Work out the finished part from the listing and answer in its coordinate system (mm). Round coordinates to 2 decimals unless told otherwise and drop trailing zeros. Order: outer loops, then holes, each group sorted by start corner. A loop starts at its lowest first (then second) coordinate and runs counter-clockwise, first axis right, second up. Notation, with made-up numbers: (-35.75, 38) - (1.25, 38) arc R31 ccw to (1.25, 70) - close; hole circle Ø10 at (74.5, 21). An arc over 180 degrees is marked (long way). Answer in a Markdown table with one row per item.
from build123d import *

# Parameters (mm, degrees)
SKETCH_1_W      = 32
SKETCH_1_H      = 10
SKETCH_1_R      = 1.25
EXTRUDE_1_DEPTH = 18
SKETCH_4_W      = 32
SKETCH_4_H      = 10
SKETCH_4_R      = 1.25
EXTRUDE_3_DEPTH = 1
FILLET_3_R      = 5
FILLET_4_R      = 5


with BuildPart() as part:
    # 草图1 → 凸台-拉伸1 (new body)
    with BuildSketch(Plane(origin=(0, 0, 0), x_dir=(1, 0, 0), z_dir=(0, 1, 0))):
        with Locations((16, 5)):
            Rectangle(SKETCH_1_W, SKETCH_1_H)
        with Locations(Location((5, 5, 0), (0, 0, 270))):
            Circle(SKETCH_1_R, mode=Mode.SUBTRACT)
        with Locations(Location((27, 5, 0), (0, 0, 270))):
            Circle(SKETCH_1_R, mode=Mode.SUBTRACT)
    extrude(amount=EXTRUDE_1_DEPTH)

    # 草图4 → 凸台-拉伸3 (add)
    with BuildSketch(Plane(origin=(0, 18, 0), x_dir=(1, 0, 0), z_dir=(0, 1, 0))):
        with Locations((16, 5)):
            Rectangle(SKETCH_4_W, SKETCH_4_H)
        with Locations(Location((5, 5, 0), (0, 0, 270))):
            Circle(SKETCH_4_R, mode=Mode.SUBTRACT)
        with Locations(Location((27, 5, 0), (0, 0, 270))):
            Circle(SKETCH_4_R, mode=Mode.SUBTRACT)
    extrude(amount=EXTRUDE_3_DEPTH)

    # 圆角3
    fillet_3_edges = [part.edges().sort_by_distance(p)[0] for p in [
        (0, 9.5, -10),
    ]]
    fillet(fillet_3_edges, radius=FILLET_3_R)

    # 圆角4
    fillet_4_edges = [part.edges().sort_by_distance(p)[0] for p in [
        (32, 9.5, -10),
        (32, 9.5, 0),
        (0, 9.5, 0),
    ]]
    fillet(fillet_4_edges, radius=FILLET_4_R - 0.0001)  # a hair under: the kernel refuses the full size


solid = part.part
1) Find section A-A, the plane y = 11.75. Give the number of separate pieces and of enclosed holes in the cut face, then the cut area to 3 significant figures.
Filled in:
| item | result |
|---|---|
| separate pieces | 1 |
| enclosed holes | 2 |
| area | 289 mm^2 |
2) This flat-tipped pin is pushed along its axis until it touches: pin 1 (1.5 mm diameter, centred on x = 27, z = -5, fed in from -Y). Where does it stop, or does it pass through?
Filled in:
| item | result |
|---|---|
| pin 1 | passes through |
3) Find section B-B, the plane z = -8.75. Give the vertices of the cut face in (x, y).
Filled in:
| item | result |
|---|---|
| outline | (1.69, 0) - (30.31, 0) - (30.31, 19) - (1.69, 19) - close |
4) Find the intervals of material crossed by probe 1 along X at (y, z) = (6.5, -5); probe 2 along X at (y, z) = (3, -5.5); probe 3 along Z at (x, y) = (27.5, 4.25), in increasing order. Write a range as from..to.
Filled in:
| item | result |
|---|---|
| probe 1 | x = 0..3.75, 6.25..25.75, 28.25..32 |
| probe 2 | x = 0.03..3.85, 6.15..25.85, 28.15..31.97 |
| probe 3 | z = -9.97..-6.15, -3.85..-0.03 |
5) The mould has two halves that part along Z. Classify faces 1 (the face through (16, 0, -5)), 2 (the face through (3.78, 9.37, -5.27)), 3 (the face through (16, 9, -10)), 4 (the face through (16, 9, 0)): released by +Z, released by -Z, zero draft, split by the parting line, or undercut.
Filled in:
| item | result |
|---|---|
| face 1 | zero draft |
| face 2 | undercut |
| face 3 | released by -Z |
| face 4 | released by +Z |
